Geometry check sheet. Reference: the model listing, model coordinates, mm. A direction names the side the tool comes from. Give positions to 0.01 mm unless a question says otherwise; leave off trailing zeros. Order: outer loops, then holes, each group sorted by start corner. A loop starts at its lowest first (then second) coordinate and runs counter-clockwise, first axis right, second up.
from build123d import *

# Parameters (mm, degrees)
SKETCH_R             = 3.175
PAD_DEPTH            = 13.462
SKETCH002_W          = 23
SKETCH002_H          = 13
POCKET_DEPTH         = 7.501
POCKET_DEPTH_BACK    = -38.001
SKETCH001_W          = 14
SKETCH001_H          = 23
POCKET001_DEPTH      = 7.501
POCKET001_DEPTH_BACK = -7.501
CHAMFER_SIZE         = 1.5
FILLET_R             = 1.016
FILLET001_R          = 1.016
CHAMFER001_SIZE      = 1
CHAMFER002_SIZE      = 1


with BuildPart() as part:
    # Sketch → Pad (new body, symmetric)
    with BuildSketch(Plane.XZ):
        with BuildLine():
            ThreePointArc((0, 7.5), (-7.5, 0), (0, -7.5))
            Line((38, -7.5), (0, -7.5))
            Line((38, 0.5), (38, -7.5))
            Line((15.5, 7.5), (38, 0.5))
            Line((0, 7.5), (15.5, 7.5))
        make_face()
        Circle(SKETCH_R, mode=Mode.SUBTRACT)
    extrude(amount=PAD_DEPTH, both=True)

    # Sketch002 → Pocket (cut, two sides)
    with BuildSketch(Plane.YZ) as pocket_sk:
        with Locations((0, 1.5)):
            Rectangle(SKETCH002_W, SKETCH002_H)
    extrude(amount=-POCKET_DEPTH, mode=Mode.SUBTRACT)
    extrude(pocket_sk.sketch, amount=-POCKET_DEPTH_BACK, mode=Mode.SUBTRACT)

    # Sketch001 → Pocket001 (cut, two sides)
    with BuildSketch(Plane.XY) as pocket001_sk:
        with Locations((-0.5, 0)):
            Rectangle(SKETCH001_W, SKETCH001_H)
        with BuildLine():
            Line((18, 2), (18, -2))
            ThreePointArc((18, -2), (20, -4), (22, -2))
            Line((22, -2), (22, 2))
            ThreePointArc((22, 2), (20, 4), (18, 2))
        make_face()
        with BuildLine():
            Line((29, 2), (29, -2))
            ThreePointArc((29, -2), (31, -4), (33, -2))
            Line((33, 2), (33, -2))
            ThreePointArc((33, 2), (31, 4), (29, 2))
        make_face()
    extrude(amount=-POCKET001_DEPTH, mode=Mode.SUBTRACT)
    extrude(pocket001_sk.sketch, amount=-POCKET001_DEPTH_BACK, mode=Mode.SUBTRACT)

    # Chamfer
    chamfer_edges = [part.edges().sort_by_distance(p)[0] for p in [
        (6.5, 0, -5),
    ]]
    chamfer(chamfer_edges, length=CHAMFER_SIZE)

    # Fillet
    fillet_edges = [part.edges().sort_by_distance(p)[0] for p in [
        (38, 12.481, 0.5),
    ]]
    fillet(fillet_edges, radius=FILLET_R)

    # Fillet001
    fillet001_edges = [part.edges().sort_by_distance(p)[0] for p in [
        (38, -12.481, 0.5),
    ]]
    fillet(fillet001_edges, radius=FILLET001_R)

    # Chamfer001
    chamfer001_edges = [part.edges().sort_by_distance(p)[0] for p in [
        (29, 0, -5),
        (31, 4, -5),
        (33, 0, -5),
        (31, -4, -5),
    ]]
    chamfer(chamfer001_edges, length=CHAMFER001_SIZE)

    # Chamfer002
    chamfer002_edges = [part.edges().sort_by_distance(p)[0] for p in [
        (22, 0, -5),
        (20, 4, -5),
        (18, 0, -5),
        (20, -4, -5),
    ]]
    chamfer(chamfer002_edges, length=CHAMFER002_SIZE)


solid = part.part
Item 1: Sectioned sample at A-A (x = 20). Enter the section's corners in (y, z).
Reported:
outline: (-13.46, -7.5) - (-4, -7.5) - (-4, -6) - (-5, -5) - (-11.5, -5) - (-11.5, 6.1) - (-13.46, 6.1) - close; (4, -7.5) - (13.46, -7.5) - (13.46, 6.1) - (11.5, 6.1) - (11.5, -5) - (5, -5) - (4, -6) - close
Item 2: Gauge pin test, flat end, axial feed: pin 1 (0.8 mm diameter, centred on y = -1, z = -7, fed in from -X). Record the tip position at first contact, or that the pin passes through.
Reported:
pin 1: stops at x = 6.5
Item 3: Set-up check for faces 1 (the flat face through (7, 0, -6)), 2 (the conical face through (31, -4.2, -5.8)), 3 (the flat face through (22, 0, -7)), 4 (the flat face through (23.2, -0.2, -5)): record each of +Z, -Z, +X, -X, +Y, -Y from which the full face is reachable in a straight line by a thin tool's end or side.
Reported:
face 1: +Z, -X
face 2: +Z
face 3: +Z, -Z
face 4: +Z, +X, -X
Item 4: Scan lines: L1, parallel to Y at x = 34, z = -4.75; L2, parallel to Z at x = 0, y = -12.6 (3 decimals); L3, parallel to Z at x = 29, y = -5.5. Record each from-to range of solid material in increasing order.
Reported:
L1: y = -13.46 to -11.5, 11.5 to 13.46
L2: z = -7.5 to -3.175, 3.175 to 7.5
L3: z = -7.5 to -5
Item 5: Sectioned sample at D-D (z = -5.5). Enter the section's corners in (x, y).
Reported:
outline: (-5.1, -13.46) - (38, -13.46) - (38, 13.46) - (-5.1, 13.46) - (-5.1, 11.5) - (7.5, 11.5) - (7.5, -11.5) - (-5.1, -11.5) - close; hole (17.5, -2) arc R2.5 ccw to (22.5, -2) - (22.5, 2) arc R2.5 ccw to (17.5, 2) - close; hole (28.5, -2) arc R2.5 ccw to (33.5, -2) - (33.5, 2) arc R2.5 ccw to (28.5, 2) - close
Item 6: Sectioned sample at C-C (z = -1.75). Enter the section's corners in (x, y), and give its area (3 significant figures).
Reported:
outline: (-7.29, -13.46) - (-2.65, -13.46) - (-2.65, -11.5) - (-7.29, -11.5) - close; (-7.29, 11.5) - (-2.65, 11.5) - (-2.65, 13.46) - (-7.29, 13.46) - close; (2.65, -13.46) - (38, -13.46) - (38, -11.5) - (2.65, -11.5) - close; (2.65, 11.5) - (38, 11.5) - (38, 13.46) - (2.65, 13.46) - close
area: 157 mm2
Item 7: Sectioned sample at B-B (y = 0.5). Enter the section's corners in (x, z), and give its area (3 significant figures).
Reported:
outline: (6.5, -7.5) - (18, -7.5) - (18, -6) - (17, -5) - (8, -5) - (6.5, -6.5) - close; (22, -7.5) - (29, -7.5) - (29, -6) - (28, -5) - (23, -5) - (22, -6) - close; (33, -7.5) - (38, -7.5) - (38, -5) - (34, -5) - (33, -6) - close
area: 55.6 mm2
